Verification items for this drawing (mm, ordinates from the low corner). Round coordinates to 2 decimals unless told otherwise and drop trailing zeros. Order: outer loops, then holes, each group sorted by start corner. A loop starts at its lowest first (then second) coordinate and runs counter-clockwise, first axis right, second up. Notation, with made-up numbers: M 82.25,-35 L 124.25,-35 A11 cw 124.25,-18 Z; hole C 77,-24.5 d7. An arc over 180 degrees is marked long. Return JSON: item names as keys, results as strings. Group by question number.
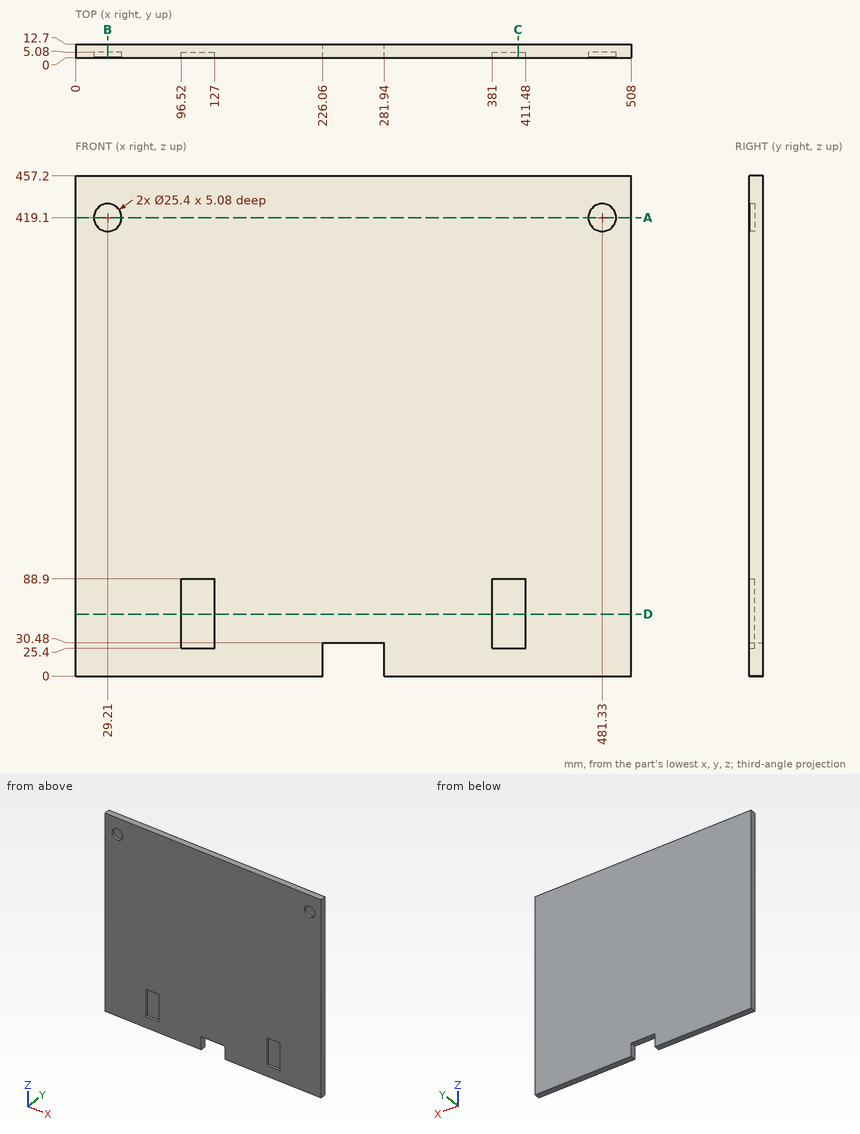
Q1. Section check D-D on z = 56.5. Record the cut outline in (x, y), plus the area to 3 significant figures.
Q2. Section check C-C on x = 404.5. Record the cut outline in (y, z), plus the area to 3 significant figures.
Q3. Material ranges on line 1 along X through (y, z) = (3.7, 419.1); line 2 along Z through (x, y) = (411, 0.5); line 3 along X through (y, z) = (2.25, 77), recorded low to high.
Q4. Section check A-A on z = 419.1. Record the cut outline in (x, y), plus the area to 3 significant figures.
Q5. Section check B-B on x = 29.21. Record the cut outline in (y, z).
Q6. Depth check by flat-ended pin: pin 1 Ø1.5 at (y, z) = (2.5, 56) entering from -X; pin 2 Ø12.5 at (x, z) = (24.5, 421.5) entering from -Y. Enter the tip coordinate at first touch or a pass-through.
Geometry check:
{
 "1": {"outline": "M 0,0 L 96.52,0 L 96.52,5.08 L 127,5.08 L 127,0 L 381,0 L 381,5.08 L 411.48,5.08 L 411.48,0 L 508,0 L 508,12.7 L 0,12.7 Z", "area": "6,140 mm^2"},
 "2": {"outline": "M 0,0 L 12.7,0 L 12.7,457.2 L 0,457.2 L 0,88.9 L 5.08,88.9 L 5.08,25.4 L 0,25.4 Z", "area": "5,480 mm^2"},
 "3": {"line 1": "x = 0 to 16.51, 41.91 to 468.63, 494.03 to 508", "line 2": "z = 0 to 25.4, 88.9 to 457.2", "line 3": "x = 0 to 96.52, 127 to 381, 411.48 to 508"},
 "4": {"outline": "M 0,0 L 16.51,0 L 16.51,5.08 L 41.91,5.08 L 41.91,0 L 468.63,0 L 468.63,5.08 L 494.03,5.08 L 494.03,0 L 508,0 L 508,12.7 L 0,12.7 Z", "area": "6,190 mm^2"},
 "5": {"outline": "M 0,0 L 12.7,0 L 12.7,457.2 L 0,457.2 L 0,431.8 L 5.08,431.8 L 5.08,406.4 L 0,406.4 Z"},
 "6": {"pin 1": "stops at x = 0", "pin 2": "stops at y = 5.08"}
}
